Answer from the drawing. Dimensions are ordinates in mm from the lowest x, y and z of the part. Coordinates: 2 decimals unless noted, no trailing zeros. Order: outer loops, then holes, each group sorted by start corner. A loop starts at its lowest first (then second) coordinate and runs counter-clockwise, first axis right, second up. Notation, with made-up numbers: (-27, 26.5) -> (1, 26.5) arc R22 cw to (1, 43.5) -> close; hole circle Ø9 at (-36, -12). An arc over 180 degrees is marked (long way). Answer as a JSON object with one key per item and string values. Group by question number.
1) Section A-A on y = 41 is taken. Determine the outline of the cut face in (x, z).
2) Consider L1, parallel to Y at x = 261, z = 16.75; L2, parallel to X at y = 67, z = 8.25. Determine where each line is inside the solid, lowest interval first.
3) Section C-C on z = 19.25 is taken. Determine the outline of the cut face in (x, y), and give its area (3 significant figures).
4) Given pin 1 (15 mm diameter, centred on x = 530.5, y = 54, fed in from -Z); pin 2 (14 mm diameter, centred on x = 180, z = 20.5, fed in from +Y); pin 3 (4 mm diameter, centred on y = 52, z = 6, fed in from +X), each flat-ended and moving along its own axis, determine where each tip first touches the part or whether it passes through.
5) Section B-B on x = 386.5 is taken. Determine the outline of the cut face in (y, z), and give its area (3 significant figures).
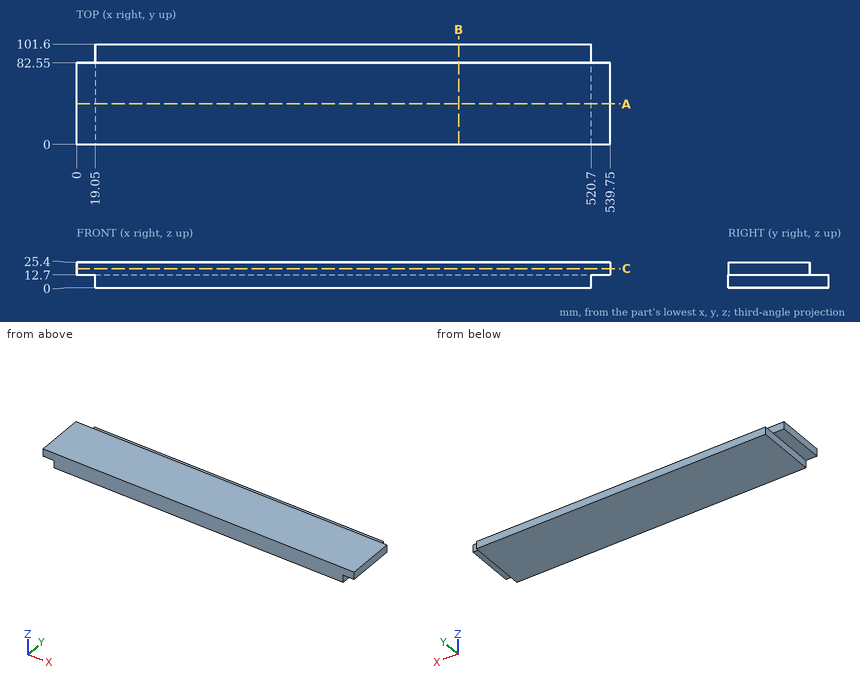
Worked answers:
{
 "1": {"outline": "(0, 12.7) -> (19.05, 12.7) -> (19.05, 0) -> (520.7, 0) -> (520.7, 12.7) -> (539.75, 12.7) -> (539.75, 25.4) -> (0, 25.4) -> close"},
 "2": {"L1": "y = 0 to 82.55", "L2": "x = 19.05 to 520.7"},
 "3": {"outline": "(0, 0) -> (539.75, 0) -> (539.75, 82.55) -> (0, 82.55) -> close", "area": "44,600 mm²"},
 "4": {"pin 1": "stops at z = 12.7", "pin 2": "stops at y = 82.55", "pin 3": "stops at x = 520.7"},
 "5": {"outline": "(0, 0) -> (101.6, 0) -> (101.6, 12.7) -> (82.55, 12.7) -> (82.55, 25.4) -> (0, 25.4) -> close", "area": "2,340 mm²"}
}
